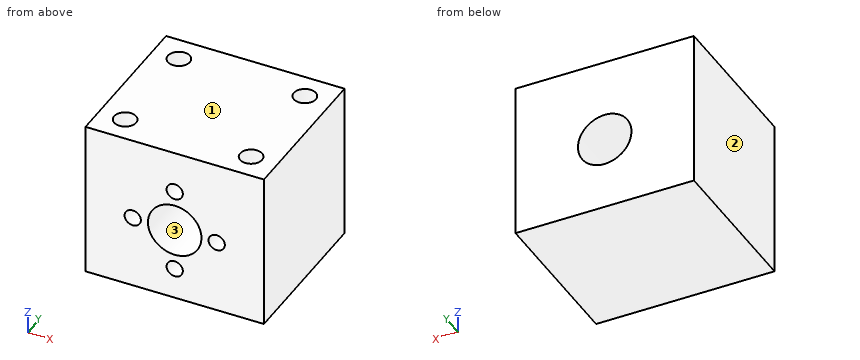
```python
from build123d import *

# Parameters (mm, degrees)
SKETCH_1_W          = 34
SKETCH_1_H          = 30
EXTRUDE_1_DEPTH     = 30
SKETCH_2_R          = 5.1
CUT_EXTRUDE_1_DEPTH = 38.603191354
SKETCH_3_R          = 1.55
CUT_EXTRUDE_2_DEPTH = 15
SKETCH_4_R          = 2.1
CUT_EXTRUDE_3_DEPTH = 20


with BuildPart() as part:
    # 草图1 → 凸台-拉伸1 (new body)
    with BuildSketch(Plane(origin=(0, 0, 0), x_dir=(1, 0, 0), z_dir=(0, 1, 0))):
        Rectangle(SKETCH_1_W, SKETCH_1_H)
    extrude(amount=EXTRUDE_1_DEPTH)

    # 草图2 → 切除-拉伸1 (cut, through all)
    with BuildSketch(Plane(origin=(0, 0, 0), x_dir=(-1, 0, 0), z_dir=(0, -1, 0))):
        with Locations(Location((0, 1, 0), (0, 0, 90))):
            Circle(SKETCH_2_R)
    extrude(amount=-CUT_EXTRUDE_1_DEPTH, mode=Mode.SUBTRACT)

    # 草图3 → 切除-拉伸2 (cut)
    with BuildSketch(Plane(origin=(0, 0, 0), x_dir=(-1, 0, 0), z_dir=(0, -1, 0))):
        with Locations(Location((8, 1, 0), (0, 0, 90))):
            Circle(SKETCH_3_R)
        with Locations(Location((0, -7, 0), (0, 0, 90))):
            Circle(SKETCH_3_R)
        with Locations(Location((-8, 1, 0), (0, 0, 90))):
            Circle(SKETCH_3_R)
        with Locations(Location((0, 9, 0), (0, 0, 90))):
            Circle(SKETCH_3_R)
    extrude(amount=-CUT_EXTRUDE_2_DEPTH, mode=Mode.SUBTRACT)

    # 草图4 → 切除-拉伸3 (cut)
    with BuildSketch(Plane.XY.offset(15)):
        with Locations((-12, 5)):
            Circle(SKETCH_4_R)
        with Locations((12, 5)):
            Circle(SKETCH_4_R)
        with Locations((12, 25)):
            Circle(SKETCH_4_R)
        with Locations((-12, 25)):
            Circle(SKETCH_4_R)
    extrude(amount=-CUT_EXTRUDE_3_DEPTH, mode=Mode.SUBTRACT)


solid = part.part
```
Build history of the part. All positions in model axes, mm. Face numbers are marked on the shaded views. Give positions to 0.01 mm unless a question says otherwise; leave off trailing zeros. Loops run counter-clockwise (first coordinate to the right, second up) from the corner with the lowest first, then second, coordinate; pieces in that order, holes last.
Item 1: Flat gauge pins, fed straight in: pin 1 (2 mm diameter, centred on x = 12, y = 4, fed in from +Z); pin 2 (1.5 mm diameter, centred on x = 7.5, z = -0.5, fed in from -Y). Where does each tip first touch, or does it go through?
Answers follow:
pin 1: stops at z = -5
pin 2: stops at y = 15
Item 2: Slice it at D-D, the plane x = -12. List the corners of the cut face in (y, z).
Answers follow:
outline: (0, -15) - (30, -15) - (30, 15) - (27.1, 15) - (27.1, -5) - (22.9, -5) - (22.9, 15) - (7.1, 15) - (7.1, -5) - (2.9, -5) - (2.9, 15) - (0, 15) - close
Item 3: Drill centre lines: line 1 (Y direction, x = 12, z = 9.75); line 2 (X direction, y = 7.25, z = -1); line 3 (X direction, y = 9.25, z = 7). Where is each one in solid material? Low to high.
Answers follow:
line 1: y = 0 to 2.9, 7.1 to 22.9, 27.1 to 30
line 2: x = -17 to -9.55, -6.45 to -5.1, 5.1 to 6.45, 9.55 to 17
line 3: x = -17 to -1.55, 1.55 to 17
Item 4: Slice it at A-A, the plane z = 3.5. List the corners of the cut face in (x, y), and give its area (3 significant figures).
Answers follow:
outline: (-17, 0) - (-2.4, 0) - (-2.4, 30) - (-17, 30) - close; (2.4, 0) - (17, 0) - (17, 30) - (2.4, 30) - close; hole circle Ø4.2 at (-12, 5); hole circle Ø4.2 at (-12, 25); hole circle Ø4.2 at (12, 5); hole circle Ø4.2 at (12, 25)
area: 821 mm2
Item 5: Slice it at B-B, the plane z = 7. List the corners of the cut face in (x, y).
Answers follow:
outline: (-17, 0) - (-1.55, 0) - (-1.55, 15) - (1.55, 15) - (1.55, 0) - (17, 0) - (17, 30) - (-17, 30) - close; hole circle Ø4.2 at (-12, 5); hole circle Ø4.2 at (-12, 25); hole circle Ø4.2 at (12, 5); hole circle Ø4.2 at (12, 25)
Item 6: Slice it at C-C, the plane y = 12.25. List the corners of the cut face in (x, z), and give its area (3 significant figures).
Answers follow:
outline: (-17, -15) - (17, -15) - (17, 15) - (-17, 15) - close; hole circle Ø3.1 at (-8, -1); hole circle Ø10.2 at (0, -1); hole circle Ø3.1 at (0, -9); hole circle Ø3.1 at (0, 7); hole circle Ø3.1 at (8, -1)
area: 908 mm2
Item 7: Pull direction Z, two halves, no side cores. Call the marked faces 1, 2 and 3: released by +Z, released by -Z, zero draft, split by the parting line, or undercut.
Answers follow:
face 1: released by +Z
face 2: zero draft
face 3: undercut
